Input: part model. Units: mm. Frame: model coordinates. Face numbers are marked on the shaded views. A direction names the side the tool comes from. Coordinates: 2 decimals unless noted, no trailing zeros. Order: outer loops, then holes, each group sorted by start corner. A loop starts at its lowest first (then second) coordinate and runs counter-clockwise, first axis right, second up. Notation, with made-up numbers: (72, -25.5) -> (104, -25.5) arc R22 cw to (104, -17.5) -> close; hole circle Ø6 at (-36.75, 28.25). An arc over 180 degrees is marked (long way). Use one line per item in the form item = value. Start each with the question number.
1) Section query D-D on y = -75. Output: boundary loops of the cut face in (x, z) (3 decimals).
2) Draft query along Y for the marked faces 4, 5 and 6. Return one class per face: pulls with the +Y half, pulls with the -Y half, needs draft (parallel to the pull), parting line crosses it, or undercut.
3) Pin query (flat end, axial travel): pin 1 (3 mm diameter, centred on x = -1.5, y = -27, fed in from +Z); pin 2 (4 mm diameter, centred on x = 6, z = -38, fed in from +Y); pin 3 (12 mm diameter, centred on x = 11, z = -36, fed in from -Y); pin 4 (8 mm diameter, centred on x = -3.5, y = -79, fed in from +Z). Return the tip coordinate at first contact, or that it passes through.
4) Section query B-B on y = 37.5. Output: boundary loops of the cut face in (x, z) (3 decimals).
5) Section query C-C on z = 15. Output: boundary loops of the cut face in (x, y) (3 decimals).
6) Access query for the marked faces 1, 2 and 3. Directions: +Z, -Z, +X, -X, +Y, -Y. A direction counts if a zero-diameter tool reaches every point of the face in a straight line with its end or side. Return the directions, or none.
7) Section query A-A on x = 6. Output: boundary loops of the cut face in (y, z), then the cut area to 3 significant figures.
8) Ray query, line 1 along Z through (x, y) = (-3.5, 4); line 2 along X through (y, z) = (-0.5, 14) (3 decimals); line 3 along Y through (x, z) = (11, 14.5). Return the intervals inside material, ascending.
from build123d import *
from build123d import SkipClean  # not in build123d's __all__

# Parameters (mm, degrees)
F1_DEPTH = 12.065
F2_R     = 38.1
F2_R_2   = 25.4
F3_DEPTH = 15.875


with BuildPart() as f1:
    # F0 (on Right) → F1 (new body, symmetric)
    with BuildSketch(Plane.YZ):
        with BuildLine():
            ThreePointArc((39.5052965482, -19.05), (34.4008644324, 0), (39.5052965482, 19.05))
            Line((39.5052965482, 19.05), (25.4080040394, 19.05))
            ThreePointArc((25.4080040394, 19.05), (21.7008644324, 0), (25.4080040394, -19.05))
            Line((25.4080040394, -19.05), (39.5052965482, -19.05))
        make_face()
        with BuildLine():
            Line((25.4080040394, 19.05), (39.5052965482, 19.05))
            ThreePointArc((39.5052965482, 19.05), (53.4508644324, 32.9955678842), (72.5008644324, 38.1))
            Line((72.5008644324, 38.1), (72.5008644324, 50.8))
            ThreePointArc((72.5008644324, 50.8), (44.1028011182, 42.1211348375), (25.4080040394, 19.05))
        make_face()
        with BuildLine():
            ThreePointArc((25.4080040394, -19.05), (21.7008644324, 0), (25.4080040394, 19.05))
            Line((25.4080040394, 19.05), (-46.9035676834, 19.05))
            ThreePointArc((-46.9035676834, 19.05), (-43.097361586, 9.8610056184), (-41.7991355676, 0))
            ThreePointArc((-41.7991355676, 0), (-43.097361586, -9.8610056184), (-46.9035676834, -19.05))
            Line((-46.9035676834, -19.05), (25.4080040394, -19.05))
        make_face()
        with BuildLine():
            ThreePointArc((72.5008644324, -38.1), (53.4508644324, -32.9955678842), (39.5052965482, -19.05))
            Line((39.5052965482, -19.05), (25.4080040394, -19.05))
            ThreePointArc((25.4080040394, -19.05), (44.1028011182, -42.1211348375), (72.5008644324, -50.8))
            Line((72.5008644324, -50.8), (72.5008644324, -38.1))
        make_face()
        with BuildLine():
            ThreePointArc((-41.7991355676, 0), (-43.097361586, 9.8610056184), (-46.9035676834, 19.05))
            Line((-46.9035676834, 19.05), (-63.0986147423, 19.05))
            ThreePointArc((-63.0986147423, 19.05), (-56.7486147423, 10.4505208253), (-54.4991355676, 0))
            ThreePointArc((-54.4991355676, 0), (-56.7486147423, -10.4505208253), (-63.0986147423, -19.05))
            Line((-63.0986147423, -19.05), (-46.9035676834, -19.05))
            ThreePointArc((-46.9035676834, -19.05), (-43.097361586, -9.8610056184), (-41.7991355676, 0))
        make_face()
        with BuildLine():
            Line((-63.0986147423, 19.05), (-46.9035676834, 19.05))
            ThreePointArc((-46.9035676834, 19.05), (-117.9991355676, 0), (-46.9035676834, -19.05))
            Line((-46.9035676834, -19.05), (-63.0986147423, -19.05))
            ThreePointArc((-63.0986147423, -19.05), (-105.2991355676, 0), (-63.0986147423, 19.05))
        make_face()
    extrude(amount=F1_DEPTH, both=True)

    # F2 (on Right) → F3 (join, symmetric)
    with BuildSketch(Plane.YZ):
        with Locations((-79.8991355676, 0)):
            Circle(F2_R)
        with Locations((-79.8991355676, 0)):
            Circle(F2_R_2, mode=Mode.SUBTRACT)
    with SkipClean():  # cleaning this boolean's faces spoils the solid; the shape is the same uncleaned
        extrude(amount=F3_DEPTH, both=True)


solid = f1.part
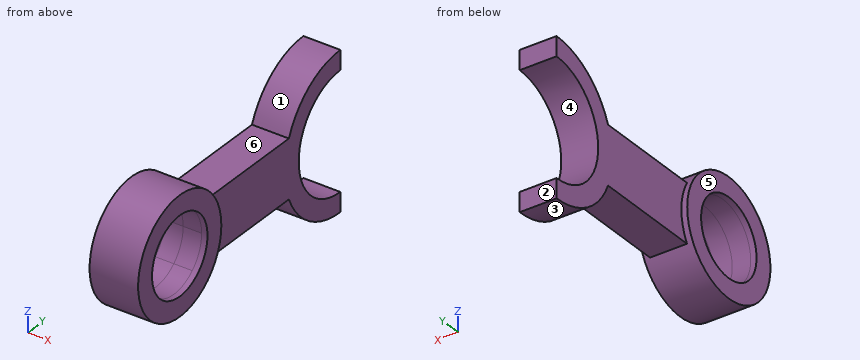
Answers below:
q1.outline = (-15.875, -37.784) -> (15.875, -37.784) -> (15.875, -24.923) -> (-15.875, -24.923) -> close; (-15.875, 24.923) -> (15.875, 24.923) -> (15.875, 37.784) -> (-15.875, 37.784) -> close
q2.face_4 = pulls with the +Y half
q2.face_5 = needs draft
q2.face_6 = undercut
q3.pin_1 = 19.05
q3.pin_2 = 72.5
q3.pin_3 = -103.39
q3.pin_4 = 38.1
q4.outline = (-12.065, -36.818) -> (12.065, -36.818) -> (12.065, -15.052) -> (-12.065, -15.052) -> close; (-12.065, 15.052) -> (12.065, 15.052) -> (12.065, 36.818) -> (-12.065, 36.818) -> close
q5.outline = (-15.875, -114.922) -> (15.875, -114.922) -> (15.875, -100.397) -> (-15.875, -100.397) -> close; (-15.875, -59.401) -> (15.875, -59.401) -> (15.875, -44.876) -> (12.065, -44.876) -> (12.065, 37.478) -> (-12.065, 37.478) -> (-12.065, -44.876) -> (-15.875, -44.876) -> close
q6.face_1 = +Z, +X, -X
q6.face_2 = +Z, -Z, +X, -X, +Y
q6.face_3 = -Z, +X, -X
q7.outline = (-46.9, -19.05) -> (25.41, -19.05) arc R50.8 ccw to (72.5, -50.8) -> (72.5, -38.1) arc R38.1 cw to (72.5, 38.1) -> (72.5, 50.8) arc R50.8 ccw to (25.41, 19.05) -> (-46.9, 19.05) arc R38.1 ccw (long way) to start; hole circle Ø50.8 at (-79.9, 0)
q7.area = 6,840 mm^2
q8.line_1 = -19.05 to 19.05
q8.line_2 = -12.065 to 12.065
q8.line_3 = -115.13 to -100.75, -59.04 to 37.27
